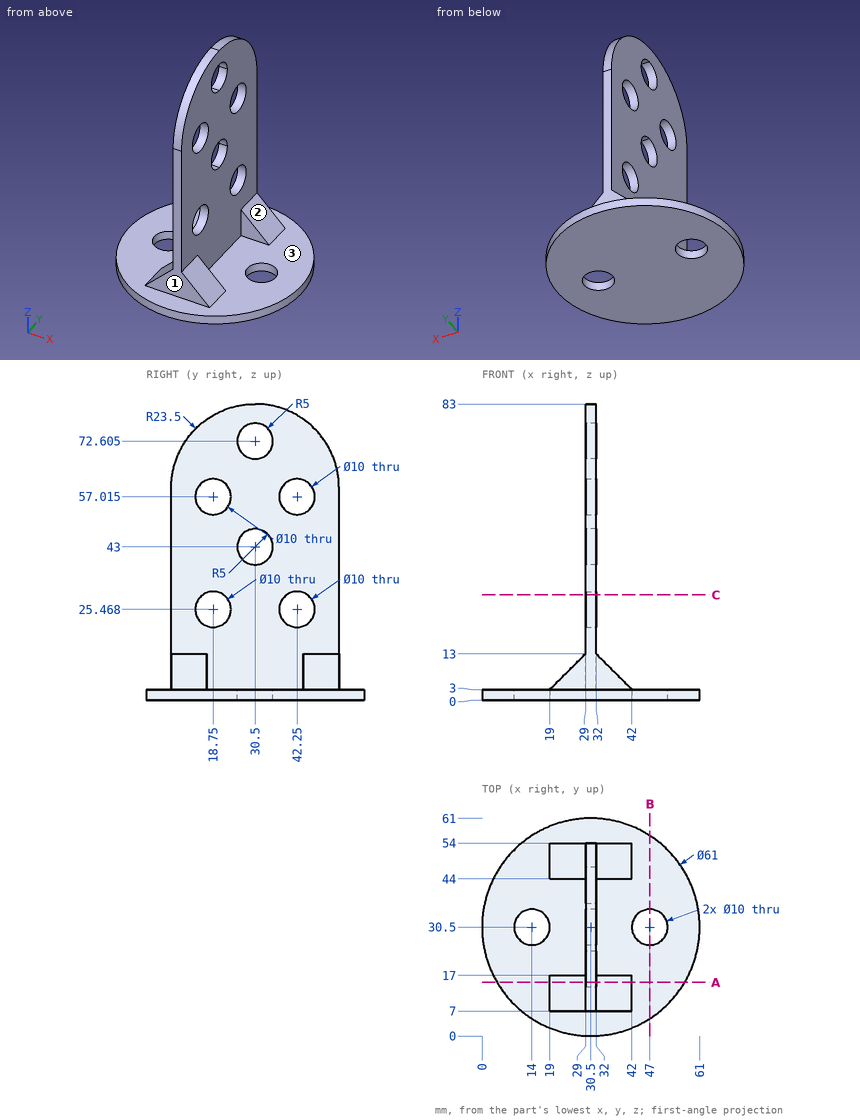
The figure shows three views and two pictorial views of one solid part (mm, origin at its lowest corner). Answer the questions. A direction names the side the tool comes from. Coordinates: 2 decimals unless noted, no trailing zeros. Loops run counter-clockwise (first coordinate to the right, second up) from the corner with the lowest first, then second, coordinate; pieces in that order, holes last.
1) Find the intervals of material crossed by L1, parallel to Y at x = 26, z = 8; L2, parallel to Y at x = 30.5, z = 60 (1 decimal); L3, parallel to X at y = 33, z = 9, in increasing order.
2) A tool of negligible diameter and unlimited length cuts with its end or side. For the marked faces 1, 2 and 3, from which of +Z, -Z, +X, -X, +Y, -Y can it reach the whole face along a straight path? Write none if from no direction.
3) Flat-ended cylindrical pins translate along their axes: pin 1 Ø12 at (y, z) = (41.5, 33.5) entering from +X; pin 2 Ø5 at (x, z) = (36, 10) entering from +Y; pin 3 Ø2 at (x, y) = (40.5, 47) entering from +Z; pin 4 Ø6 at (y, z) = (18.75, 25.47) entering from -X. Find the tip coordinate at first contact, or state that the pin passes through.
4) Find section B-B on x = 47. Write down the section's boundary in (y, z).
5) Find section A-A on y = 15. Give the number of separate pieces and of enclosed holes in the cut face.
6) Find section C-C on z = 29.5. Write down the section's boundary in (x, y).
Values:
1. L1: y = 7 to 17, 44 to 54
1. L2: y = 7 to 14.7, 22.8 to 38.2, 46.3 to 54
1. L3: x = 29 to 32
2. face 1: +Z, +X, -X, -Y
2. face 2: +Z, +X, +Y, -Y
2. face 3: +Z
3. pin 1: stops at x = 32
3. pin 2: stops at y = 54
3. pin 3: stops at z = 5.5
3. pin 4: passes through
4. outline: (4.85, 0) - (25.5, 0) - (25.5, 3) - (4.85, 3) - close; (35.5, 0) - (56.15, 0) - (56.15, 3) - (35.5, 3) - close
5. separate pieces: 3
5. enclosed holes: 0
6. outline: (29, 7) - (32, 7) - (32, 15.79) - (29, 15.79) - close; (29, 21.71) - (32, 21.71) - (32, 39.29) - (29, 39.29) - close; (29, 45.21) - (32, 45.21) - (32, 54) - (29, 54) - close
